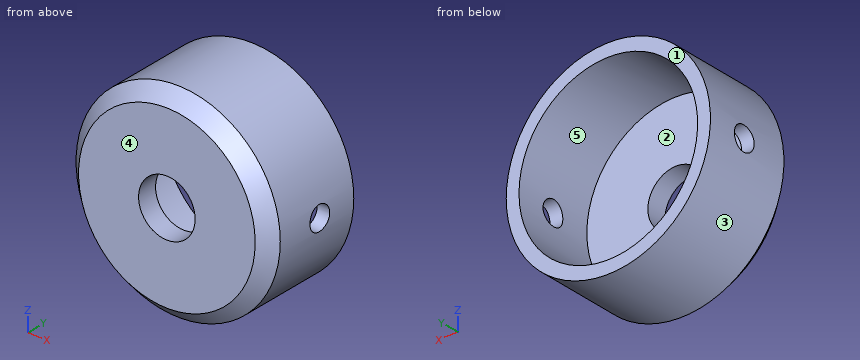
from build123d import *

# Parameters (mm, degrees)
SKETCH1_R               = 14.8
BOSS_EXTRUDE1_DEPTH     = 15
SKETCH2_R               = 12.95
CUT_EXTRUDE1_DEPTH      = 12
SKETCH3_R               = 1.75
CUT_EXTRUDE2_DEPTH      = 15.8
CUT_EXTRUDE2_DEPTH_BACK = 15.8
SKETCH4_R               = 4.1
CUT_EXTRUDE3_DEPTH      = 16.0000001
CHAMFER1_SIZE           = 2


with BuildPart() as part:
    # Sketch1 → Boss-Extrude1 (new body)
    with BuildSketch(Plane(origin=(0, 0, 0), x_dir=(1, 0, 0), z_dir=(0, 1, 0))):
        Circle(SKETCH1_R)
    extrude(amount=BOSS_EXTRUDE1_DEPTH)

    # Sketch2 → Cut-Extrude1 (cut)
    with BuildSketch(Plane(origin=(0, 15, 0), x_dir=(1, 0, 0), z_dir=(0, 1, 0))):
        Circle(SKETCH2_R)
    extrude(amount=-CUT_EXTRUDE1_DEPTH, mode=Mode.SUBTRACT)

    # Sketch3 → Cut-Extrude2 (cut, two sides)
    with BuildSketch(Plane(origin=(0, 0, 0), x_dir=(0, 0, -1), z_dir=(1, 0, 0))) as cut_extrude2_sk:
        with Locations((0, 9)):
            Circle(SKETCH3_R)
    extrude(amount=CUT_EXTRUDE2_DEPTH, mode=Mode.SUBTRACT)
    extrude(cut_extrude2_sk.sketch, amount=-CUT_EXTRUDE2_DEPTH_BACK, mode=Mode.SUBTRACT)

    # Sketch4 → Cut-Extrude3 (cut, through all)
    with BuildSketch(Plane.XZ):
        Circle(SKETCH4_R)
    extrude(amount=-CUT_EXTRUDE3_DEPTH, mode=Mode.SUBTRACT)

    # Chamfer1
    chamfer1_edges = [part.edges().sort_by_distance(p)[0] for p in [
        (-14.8, 0, 0),
    ]]
    chamfer(chamfer1_edges, length=CHAMFER1_SIZE)


solid = part.part
Read the model definition and answer for the solid it produces. Units are mm, in the model's axes. Face numbers are marked on the shaded views. A direction names the side the tool comes from. Give positions to 0.01 mm unless a question says otherwise; leave off trailing zeros. Loops run counter-clockwise (first coordinate to the right, second up) from the corner with the lowest first, then second, coordinate; pieces in that order, holes last. Notation, with made-up numbers: (51, -29.5) -> (55, -29.5) arc R19 cw to (55, -15.5) -> close; hole circle Ø1 at (11, 56.5). An arc over 180 degrees is marked (long way). Use a Markdown table: item, result.
Q1. Section B-B, the plane z = 0 is taken. Determine the outline of the cut face in (x, y).
Solved:
| item | result |
|---|---|
| outline | (-14.8, 2) -> (-12.8, 0) -> (-4.1, 0) -> (-4.1, 3) -> (-12.95, 3) -> (-12.95, 7.25) -> (-14.8, 7.25) -> close; (-14.8, 10.75) -> (-12.95, 10.75) -> (-12.95, 15) -> (-14.8, 15) -> close; (4.1, 0) -> (12.8, 0) -> (14.8, 2) -> (14.8, 7.25) -> (12.95, 7.25) -> (12.95, 3) -> (4.1, 3) -> close; (12.95, 10.75) -> (14.8, 10.75) -> (14.8, 15) -> (12.95, 15) -> close |
Q2. Each of these flat-tipped pins is pushed along its axis until it touches: pin 1 (2 mm diameter, centred on y = 12, z = 3.5, fed in from -X); pin 2 (3 mm diameter, centred on x = -8.5, y = 12.5, fed in from -Z); pin 3 (4 mm diameter, centred on x = -10.5, y = 10, fed in from -Z). Where does it stop, or does it pass through?
Solved:
| item | result |
|---|---|
| pin 1 | stops at x = -14.59 |
| pin 2 | stops at z = -13.04 |
| pin 3 | stops at z = -12.12 |
Q3. Find the intervals of material crossed by line 1 along X through (y, z) = (11.75, 0); line 2 along Y through (x, z) = (-7.25, -2), in increasing order.
Solved:
| item | result |
|---|---|
| line 1 | x = -14.8 to -12.95, 12.95 to 14.8 |
| line 2 | y = 0 to 3 |
Q4. Section D-D, the plane y = 4 is taken. Determine the outline of the cut face in (x, z), then the cut area to 3 significant figures.
Solved:
| item | result |
|---|---|
| outline | circle Ø29.6 at (0, 0); hole circle Ø25.9 at (0, 0) |
| area | 161 mm^2 |
Q5. Determine the mould class of the marked faces 3, 4 and 5 for opening direction X: pulls with the +X half, pulls with the -X half, needs draft (parallel to the pull), parting line crosses it, or undercut.
Solved:
| item | result |
|---|---|
| face 3 | parting line crosses it |
| face 4 | needs draft |
| face 5 | undercut |
Q6. Section A-A, the plane x = 0 is taken. Determine the outline of the cut face in (y, z).
Solved:
| item | result |
|---|---|
| outline | (0, -12.8) -> (2, -14.8) -> (15, -14.8) -> (15, -12.95) -> (3, -12.95) -> (3, -4.1) -> (0, -4.1) -> close; (0, 4.1) -> (3, 4.1) -> (3, 12.95) -> (15, 12.95) -> (15, 14.8) -> (2, 14.8) -> (0, 12.8) -> close |
Q7. A tool of negligible diameter and unlimited length cuts with its end or side. For the marked faces 1 and 2, from which of +Z, -Z, +X, -X, +Y, -Y can it reach the whole face along a straight path? Write none if from no direction.
Solved:
| item | result |
|---|---|
| face 1 | +Z, -Z, +X, -X, +Y |
| face 2 | +Y |
